Input: part model. Units: mm. Frame: model coordinates. A direction names the side the tool comes from. Round coordinates to 2 decimals unless told otherwise and drop trailing zeros. Loops run counter-clockwise (first coordinate to the right, second up) from the corner with the lowest first, then second, coordinate; pieces in that order, holes last.
(1) Line query: line 1 (X direction, y = 0.25, z = 0); line 2 (X direction, y = 4.1, z = 0); line 3 (Y direction, x = -42, z = -13.5). Output: solid intervals per line, ascending.
(2) Cut plane A-A, the plane y = -1.25. Output: boundary loops of the cut face in (x, z).
(3) Cut plane C-C, the plane z = -13. Output: boundary loops of the cut face in (x, y), and give its area (3 significant figures).
(4) Cut plane B-B, the plane z = 0. Output: boundary loops of the cut face in (x, y), and give its area (3 significant figures).
(5) First-contact query: pin 1 Ø3.5 at (x, z) = (0, 0) entering from -Y; pin 2 Ø1.5 at (y, z) = (2, 3.5) entering from +X; pin 3 Ø5 at (x, y) = (-15.5, 2) entering from -Z; pin 4 Ø2 at (x, y) = (-26, 3) entering from -Z. Flat tips, straight axial feed; report the tip coordinate or a pass-through.
(6) Access query for faces 1 (the face through (-7.81, 3.27, -1.73)), 2 (the face through (-28.14, 0.03, 2.2)), 3 (the face through (-40, -2, -1)). Directions: +Z, -Z, +X, -X, +Y, -Y. A direction counts if a zero-diameter tool reaches every point of the face in a straight line with its end or side. Return the directions, or none.
(7) Cut plane D-D, the plane z = -9. Output: boundary loops of the cut face in (x, y), and give its area (3 significant figures).
(8) Draft query along Y for faces 4 (the face through (-36, 4.75, -1)), 5 (the face through (-27, -4.75, -1)), 6 (the face through (-13, 0, -10.5)), 7 (the face through (-45.927, 0.028, 3.228)). Return one class per face: released by +Y, released by -Y, zero draft, split by the parting line, or undercut.
from build123d import *

# Parameters (mm, degrees)
SKETCH1_R                       = 2
BOSS_EXTRUDE1_DEPTH             = 4.75
CUT_EXTRUDE1_DEPTH              = 2
BOSS_EXTRUDE2_REACH             = 69.423
BOSS_EXTRUDE2_DIRECTION_2_REACH = 69.423
CUT_EXTRUDE2_DEPTH              = 2
SKETCH7_R                       = 8
CUT_EXTRUDE3_DEPTH              = 3


with BuildPart() as part:
    # Sketch1 → Boss-Extrude1 (new, symmetric)
    with BuildSketch(Plane(origin=(0, 0, 0), x_dir=(1, 0, 0), z_dir=(0, 1, 0))):
        with BuildLine():
            Line((0, -10.500399217), (-55.93053828, -10.500399217))
            ThreePointArc((-55.93053828, -10.500399217), (-66.430937497, 0), (-55.93053828, 10.500399217))
            Line((-55.93053828, 10.500399217), (0, 10.500399217))
            ThreePointArc((0, 10.500399217), (10.500399217, 0), (0, -10.500399217))
        make_face()
        with Locations(Location((0, 0, 0), (0, 0, 270))):
            Circle(SKETCH1_R, mode=Mode.SUBTRACT)
        with Locations(Location((-55.93053828, 0, 0), (0, 0, 270))):
            Circle(SKETCH1_R, mode=Mode.SUBTRACT)
    extrude(amount=BOSS_EXTRUDE1_DEPTH, both=True)

    # Sketch3 → Cut-Extrude1 (cut, symmetric)
    with BuildSketch(Plane(origin=(0, 0, 0), x_dir=(1, 0, 0), z_dir=(0, 1, 0))):
        with BuildLine():
            Line((-35.751827911, 18.875253657), (-39.299525946, 5.868950542))
            Line((-39.299525946, 5.868950542), (26.645239155, -41.810424095))
            ThreePointArc((26.645239155, -41.810424095), (-18.563858299, -45.972421055), (-48.206523525, -11.584965354))
            Line((-48.206523525, -11.584965354), (-43.887265107, 4.249974277))
            Line((-43.887265107, 4.249974277), (-54.812276631, 12.148974547))
            ThreePointArc((-54.812276631, 12.148974547), (-46.585078234, 19.204535889), (-35.751827911, 18.875253657))
        make_face()
    extrude(amount=CUT_EXTRUDE1_DEPTH, both=True, mode=Mode.SUBTRACT)

    # Boss-Extrude2: up to this face of the body (flat: up to its plane)
    boss_extrude2_end = Plane(part.part.faces().sort_by_distance((-27.96526914, 4.75, 0))[0])
    # Sketch5 → Boss-Extrude2 (add, up to the picked face)
    with BuildSketch(Plane(origin=(0, 0, 0), x_dir=(1, 0, 0), z_dir=(0, 1, 0)), mode=Mode.PRIVATE) as boss_extrude2_sk1:
        with BuildLine():
            ThreePointArc((-24.917700351, 10.500399217), (-40.424119316, 19.553005923), (-55.93053828, 10.500399217))
            Line((-55.93053828, 10.500399217), (-24.917700351, 10.500399217))
        make_face()
    boss_extrude2_tool1 = split(extrude(boss_extrude2_sk1.sketch, amount=BOSS_EXTRUDE2_REACH, mode=Mode.PRIVATE), bisect_by=boss_extrude2_end, keep=Keep.BOTH, mode=Mode.PRIVATE)
    add(boss_extrude2_tool1.solids().sort_by(Axis((-40.424119, 0, -14.214125), (0, 1, 0)))[0])

    # Boss-Extrude2 direction 2: up to this face of the body (flat: up to its plane)
    boss_extrude2_direction_2_end = Plane(part.part.faces().sort_by_distance((-27.96526914, -4.75, 0))[0])
    # Sketch5 → Boss-Extrude2 direction 2 (add, up to the picked face)
    with BuildSketch(Plane(origin=(0, 0, 0), x_dir=(1, 0, 0), z_dir=(0, 1, 0)), mode=Mode.PRIVATE) as boss_extrude2_direction_2_sk1:
        with BuildLine():
            ThreePointArc((-24.917700351, 10.500399217), (-40.424119316, 19.553005923), (-55.93053828, 10.500399217))
            Line((-55.93053828, 10.500399217), (-24.917700351, 10.500399217))
        make_face()
    boss_extrude2_direction_2_tool1 = split(extrude(boss_extrude2_direction_2_sk1.sketch, amount=-BOSS_EXTRUDE2_DIRECTION_2_REACH, mode=Mode.PRIVATE), bisect_by=boss_extrude2_direction_2_end, keep=Keep.BOTH, mode=Mode.PRIVATE)
    add(boss_extrude2_direction_2_tool1.solids().sort_by(Axis((-40.424119, 0, -14.214125), (0, -1, 0)))[0])

    # Sketch6 → Cut-Extrude2 (cut, symmetric)
    with BuildSketch(Plane(origin=(0, 0, 0), x_dir=(1, 0, 0), z_dir=(0, 1, 0))):
        with BuildLine():
            Line((-39.299525946, 5.868950542), (-16.659276721, -10.500399217))
            Line((-16.659276721, -10.500399217), (-47.910689027, -10.500399217))
            Line((-47.910689027, -10.500399217), (-43.887265107, 4.249974277))
            Line((-43.887265107, 4.249974277), (-54.854382526, 12.179417945))
            ThreePointArc((-54.854382526, 12.179417945), (-46.349897212, 18.538096729), (-35.738154791, 18.925381021))
            Line((-35.738154791, 18.925381021), (-39.299525946, 5.868950542))
        make_face()
    extrude(amount=CUT_EXTRUDE2_DEPTH, both=True, mode=Mode.SUBTRACT)

    # Sketch7 → Cut-Extrude3 (cut)
    with BuildSketch(Plane(origin=(0, 4.75, 0), x_dir=(1, 0, 0), z_dir=(0, 1, 0))):
        with Locations(Location((0, 0, 0), (0, 0, 270))):
            Circle(SKETCH7_R)
    extrude(amount=-CUT_EXTRUDE3_DEPTH, mode=Mode.SUBTRACT)


solid = part.part
Reported:
1. line 1: x = -66.43 to -57.93, -53.93 to -45.05, -31.18 to -2, 2 to 10.5
1. line 2: x = -66.43 to -57.93, -53.93 to -8, 8 to 10.5
1. line 3: y = -4.75 to -2, 2 to 4.75
2. outline: (-55.93, -10.5) arc R17.81 ccw to (-54.85, -12.18) - (-43.89, -4.25) - (-47.91, 10.5) - (-55.93, 10.5) arc R10.5 ccw to start; (-39.3, -5.87) - (-35.74, -18.93) arc R17.81 ccw to (-24.92, -10.5) - (0, -10.5) arc R10.5 ccw to (0, 10.5) - (-16.66, 10.5) - close; hole circle Ø4 at (-55.93, 0); hole circle Ø4 at (0, 0)
3. outline: (-54.22, -4.75) - (-26.62, -4.75) - (-26.62, 4.75) - (-54.22, 4.75) - (-54.22, 2) - (-37.35, 2) - (-37.35, -2) - (-54.22, -2) - close
3. area: 195 mm2
4. outline: (-66.43, -4.75) - (-57.93, -4.75) - (-57.93, 4.75) - (-66.43, 4.75) - close; (-53.93, -4.75) - (-2, -4.75) - (-2, 1.75) - (-8, 1.75) - (-8, 4.75) - (-53.93, 4.75) - close; (2, -4.75) - (10.5, -4.75) - (10.5, 4.75) - (8, 4.75) - (8, 1.75) - (2, 1.75) - close; hole (-45.05, -2) - (-31.18, -2) - (-31.18, 2) - (-45.05, 2) - close
4. area: 563 mm2
5. pin 1: passes through
5. pin 2: stops at x = 10.13
5. pin 3: stops at z = -10.5
5. pin 4: stops at z = -13.45
6. face 1: +Y
6. face 2: +Z
6. face 3: none
7. outline: (-61.34, -4.75) - (5.41, -4.75) - (5.41, 4.75) - (-61.34, 4.75) - close; hole (-50.46, -2) - (-38.45, -2) - (-38.45, 2) - (-50.46, 2) - close
7. area: 586 mm2
8. face 4: released by +Y
8. face 5: released by -Y
8. face 6: zero draft
8. face 7: undercut
